Answer from the drawing. Dimensions are ordinates in mm from the lowest x, y and z of the part. Round coordinates to 2 decimals unless told otherwise and drop trailing zeros. Loops run counter-clockwise (first coordinate to the right, second up) from the corner with the lowest first, then second, coordinate; pieces in that order, holes last.
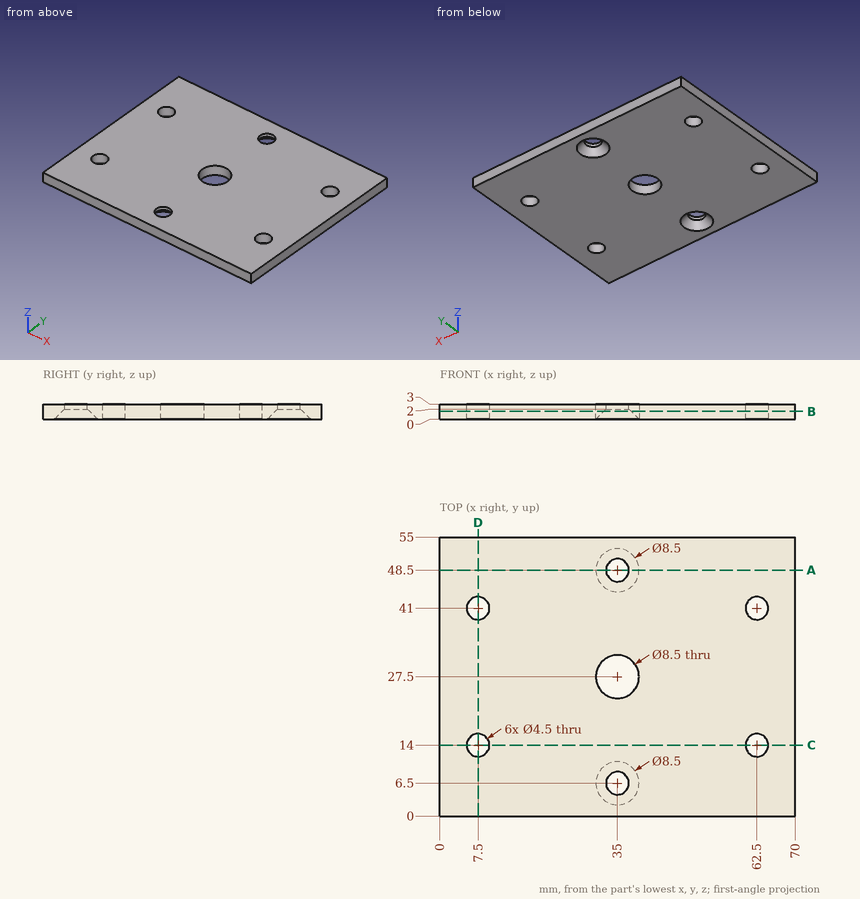
1. Find section C-C (y = 14). Write down the section's boundary in (x, z), then the cut area to 3 significant figures.
Answer key:
outline: (0, 0) - (5.25, 0) - (5.25, 3) - (0, 3) - close; (9.75, 0) - (60.25, 0) - (60.25, 3) - (9.75, 3) - close; (64.75, 0) - (70, 0) - (70, 3) - (64.75, 3) - close
area: 183 mm2
2. Consider probe 1 along Y at (x, z) = (35, 2.75); probe 2 along Y at (x, z) = (7.5, 2.45); probe 3 along X at (y, z) = (48.5, 2.55). Determine where each line is inside the solid, lowest interval first.
Answer key:
probe 1: y = 0 to 4.25, 8.75 to 23.25, 31.75 to 46.25, 50.75 to 55
probe 2: y = 0 to 11.75, 16.25 to 38.75, 43.25 to 55
probe 3: x = 0 to 32.75, 37.25 to 70
3. Find section B-B (z = 1.55). Write down the section's boundary in (x, y), then the cut area to 3 significant figures.
Answer key:
outline: (0, 0) - (70, 0) - (70, 55) - (0, 55) - close; hole circle Ø4.5 at (7.5, 14); hole circle Ø4.5 at (7.5, 41); hole circle Ø8.5 at (35, 27.5); hole circle Ø5.4 at (35, 6.5); hole circle Ø5.4 at (35, 48.5); hole circle Ø4.5 at (62.5, 14); hole circle Ø4.5 at (62.5, 41)
area: 3,680 mm2
4. Find section A-A (y = 48.5). Write down the section's boundary in (x, z).
Answer key:
outline: (0, 0) - (30.75, 0) - (32.75, 2) - (32.75, 3) - (0, 3) - close; (37.25, 2) - (39.25, 0) - (70, 0) - (70, 3) - (37.25, 3) - close
5. Find section D-D (x = 7.5). Write down the section's boundary in (y, z).
Answer key:
outline: (0, 0) - (11.75, 0) - (11.75, 3) - (0, 3) - close; (16.25, 0) - (38.75, 0) - (38.75, 3) - (16.25, 3) - close; (43.25, 0) - (55, 0) - (55, 3) - (43.25, 3) - close
6. Given pin 1 (7 mm diameter, centred on x = 7.5, y = 41, fed in from +Z); pin 2 (3.5 mm diameter, centred on x = 62.5, y = 41, fed in from -Z), each flat-ended and moving along its own axis, determine where each tip first touches the part or whether it passes through.
Answer key:
pin 1: stops at z = 3
pin 2: passes through
